Geometry check sheet. Reference: drawing and pictorial views, mm from the part's lowest x, y, z. A direction names the side the tool comes from. Give positions to 0.01 mm unless a question says otherwise; leave off trailing zeros. Order: outer loops, then holes, each group sorted by start corner. A loop starts at its lowest first (then second) coordinate and runs counter-clockwise, first axis right, second up. Notation, with made-up numbers: (72.5, 48.5) -> (100.5, 48.5) arc R33 cw to (100.5, 84.5) -> close; hole circle Ø5 at (-5.75, 58.25). An arc over 180 degrees is marked (long way). Write each question's results on one line, items separated by ' | '. Start each with the question number.
1. Depth check by flat-ended pin: pin 1 Ø10 at (y, z) = (16, 55) entering from -X; pin 2 Ø7.5 at (x, y) = (179, 13.5) entering from +Z; pin 3 Ø8 at (y, z) = (21.5, 91) entering from -X. Enter the tip coordinate at first touch or a pass-through.
2. Material ranges on L1, parallel to X at y = 5.25, z = 47 (1 decimal); L2, parallel to X at y = 15.25, z = 22.5 (1 decimal); L3, parallel to Z at x = 32.5, y = 8.75 (1 decimal), recorded low to high. Write a range as from..to.
3. Set-up check for the marked faces 1, 2 and 3: record each of +Z, -Z, +X, -X, +Y, -Y from which the full face is reachable in a straight line by a thin tool's end or side.
4. Cross-section at D-D, the plane z = 104. Enter the section's corners in (x, y) (1 decimal), then the cut area to 3 significant figures.
5. Cross-section at C-C, the plane x = 98.5. Enter the section's corners in (y, z), then the cut area to 3 significant figures.
6. Cross-section at B-B, the plane z = 58. Enter the section's corners in (x, y), then the cut area to 3 significant figures.
7. Mould release check, pull along Z, two halves, no side actions. Record for the marked faces 4, 5 and 6: +Z half, -Z half, draft (parallel to the pull), parting line (faces both ways), or undercut.
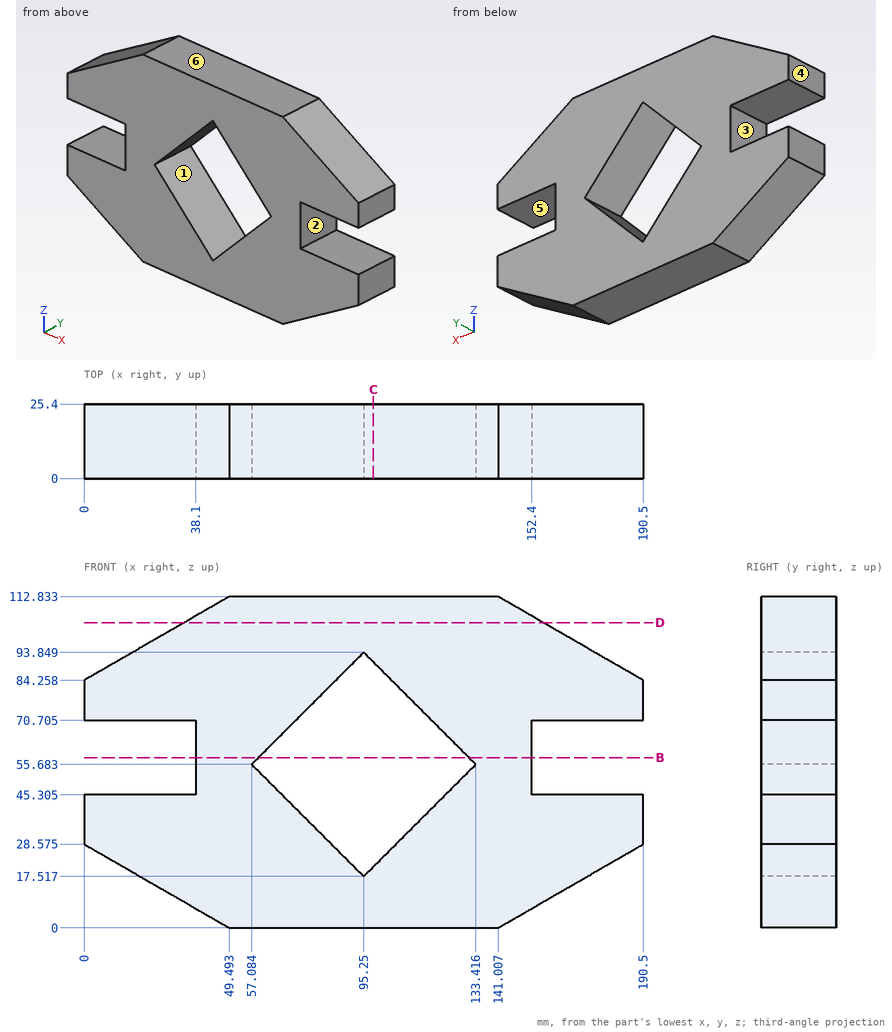
Results below:
1) pin 1: stops at x = 38.1 | pin 2: stops at z = 93.06 | pin 3: stops at x = 4.75
2) L1: x = 38.1..65.8, 124.7..152.4 | L2: x = 10.5..90.3, 100.2..180 | L3: z = 9.8..45.3, 70.7..103
3) face 1: +Y, -Y | face 2: +X, +Y, -Y | face 3: -X, +Y, -Y
4) outline: (34.2, 0) -> (156.3, 0) -> (156.3, 25.4) -> (34.2, 25.4) -> close | area: 3,100 mm²
5) outline: (0, 0) -> (25.4, 0) -> (25.4, 20.77) -> (0, 20.77) -> close; (0, 90.6) -> (25.4, 90.6) -> (25.4, 112.83) -> (0, 112.83) -> close | area: 1,090 mm²
6) outline: (38.1, 0) -> (59.4, 0) -> (59.4, 25.4) -> (38.1, 25.4) -> close; (131.1, 0) -> (152.4, 0) -> (152.4, 25.4) -> (131.1, 25.4) -> close | area: 1,080 mm²
7) face 4: draft | face 5: undercut | face 6: +Z half
